Verification items for the finished model (mm, model axes). A direction names the side the tool comes from. Coordinates: 2 decimals unless noted, no trailing zeros. Order: outer loops, then holes, each group sorted by start corner. A loop starts at its lowest first (then second) coordinate and runs counter-clockwise, first axis right, second up. Notation, with made-up numbers: M 51,75 L 80,75 A22 cw 80,110 Z; hole C 63,8 d6. An arc over 180 degrees is marked long. Return JSON: item names as keys, results as strings. Group by question number.
Q1. Section check B-B, the plane y = 0. Enter the section's corners in (x, z).
Q2. Section check A-A, the plane x = 16. Enter the section's corners in (y, z), then the cut area to 3 significant figures.
Q3. Section check C-C, the plane z = 2.5. Enter the section's corners in (x, y), then the cut area to 3 significant figures.
Q4. Go/stop test with flat-tipped pins: pin 1 Ø4 at (x, y) = (10.5, -2) entering from -Z; pin 2 Ø2 at (y, z) = (-2.5, 10.5) entering from +X; pin 3 Ø1 at (x, z) = (22, 1) entering from +Y; pin 4 Ø1.8 at (y, z) = (2, 7.5) entering from -X. Record where each tip stops, or that it passes through.
Q5. Section check D-D, the plane x = -1. Enter the section's corners in (y, z).
Q6. Thickness scan on probe 1 along Z at (x, y) = (16, -3.25); probe 2 along Y at (x, z) = (20, 1.6); probe 3 along X at (y, z) = (2, 11). Record the ranges inside material, lowest first.
Q7. Mould release check, pull along X, two halves, no side actions. Record for faces 1 (the face through (25.5, 0.1, 10.5)), 2 (the face through (3, 0, 3)), 3 (the face through (-0.54, -2.44, 10.48)): pulls with the +X half, pulls with the -X half, needs draft (parallel to the pull), parting line crosses it, or undercut.
Q8. Access from +Z, -Z, +X, -X, +Y, -Y to the whole of each face (thin tool, end or side, straight path). Record for faces 4 (the face through (7, 0, 6)), 5 (the face through (13, 0, 6)), 6 (the face through (-0.54, -2.44, 1.48)).
from build123d import *

# Parameters (mm, degrees)
BOSS_EXTRUDE1_DEPTH = 12
SKETCH6_W           = 12.5
SKETCH6_H           = 6
CUT_EXTRUDE1_DEPTH  = 31.253099015
SKETCH2_R           = 2.5
CUT_EXTRUDE2_DEPTH  = 29.714108031


with BuildPart() as part:
    # Sketch5 → Boss-Extrude1 (new body)
    with BuildSketch(Plane.XY):
        with BuildLine():
            Line((0, 5.5), (20, 5.5))
            ThreePointArc((20, 5.5), (25.5, 0), (20, -5.5))
            Line((20, -5.5), (0, -5.5))
            ThreePointArc((0, -5.5), (-5.5, 0), (0, 5.5))
        make_face()
    extrude(amount=BOSS_EXTRUDE1_DEPTH)

    # Sketch6 → Cut-Extrude1 (cut, through all)
    with BuildSketch(Plane(origin=(0, 5.5, 0), x_dir=(1, 0, 0), z_dir=(0, 1, 0))):
        with Locations((0.75, -6)):
            Rectangle(SKETCH6_W, SKETCH6_H)
        with Locations((19.25, -6)):
            Rectangle(SKETCH6_W, SKETCH6_H)
    extrude(amount=-CUT_EXTRUDE1_DEPTH, mode=Mode.SUBTRACT)

    # Sketch2 → Cut-Extrude2 (cut, through all)
    with BuildSketch(Plane.XY):
        Circle(SKETCH2_R)
        with Locations(Location((20, 0, 0), (0, 0, 180))):
            Circle(SKETCH2_R)
    extrude(amount=CUT_EXTRUDE2_DEPTH, mode=Mode.SUBTRACT)


solid = part.part
Numbers:
{
 "1": {"outline": "M -5.5,0 L -2.5,0 L -2.5,3 L -5.5,3 Z; M -5.5,9 L -2.5,9 L -2.5,12 L -5.5,12 Z; M 2.5,0 L 17.5,0 L 17.5,3 L 13,3 L 13,9 L 17.5,9 L 17.5,12 L 2.5,12 L 2.5,9 L 7,9 L 7,3 L 2.5,3 Z; M 22.5,0 L 25.5,0 L 25.5,3 L 22.5,3 Z; M 22.5,9 L 25.5,9 L 25.5,12 L 22.5,12 Z"},
 "2": {"outline": "M -5.5,0 L 5.5,0 L 5.5,3 L -5.5,3 Z; M -5.5,9 L 5.5,9 L 5.5,12 L -5.5,12 Z", "area": "66.0 mm2"},
 "3": {"outline": "M 0,-5.5 L 20,-5.5 A5.5 ccw 20,5.5 L 0,5.5 A5.5 ccw Z; hole C 0,0 d5; hole C 20,0 d5", "area": "276 mm2"},
 "4": {"pin 1": "stops at z = 0", "pin 2": "stops at x = 25.29", "pin 3": "stops at y = 5.29", "pin 4": "stops at x = 7"},
 "5": {"outline": "M -5.41,0 L -2.29,0 L -2.29,3 L -5.41,3 Z; M -5.41,9 L -2.29,9 L -2.29,12 L -5.41,12 Z; M 2.29,0 L 5.41,0 L 5.41,3 L 2.29,3 Z; M 2.29,9 L 5.41,9 L 5.41,12 L 2.29,12 Z"},
 "6": {"probe 1": "z = 0 to 3, 9 to 12", "probe 2": "y = -5.5 to -2.5, 2.5 to 5.5", "probe 3": "x = -5.12 to -1.5, 1.5 to 18.5, 21.5 to 25.12"},
 "7": {"face 1": "pulls with the +X half", "face 2": "needs draft", "face 3": "undercut"},
 "8": {"face 4": "-X, +Y, -Y", "face 5": "+X, +Y, -Y", "face 6": "+Z, -Z"}
}
